```python
from build123d import *

# Parameters (mm, degrees)
F0_R     = 11.1125
F1_DEPTH = 62.0559846
F2_R     = 2.15265
F3_DEPTH = 6.35
F4_W     = 0.635
F4_H     = 0.635
F6_R     = 11.7475
F6_R_2   = 11.1125
F7_DEPTH = 0.635


# Not quite as in the source:
# - an extrude ends at something that could not be found from the text; its depth is read off the source's solid


with BuildPart() as f1:
    # F0 (on Top) → F1 (new body)
    with BuildSketch(Plane.XY):
        with BuildLine():
            ThreePointArc((14.2875, 0), (0, 14.2875), (-14.2875, 0))
            Line((-14.2875, 0), (-14.2875, -7.9375))
            Line((-14.2875, -7.9375), (-23.8125, -7.9375))
            Line((-23.8125, -7.9375), (-23.8125, -14.2875))
            Line((-23.8125, -14.2875), (23.8125, -14.2875))
            Line((23.8125, -14.2875), (23.8125, -7.9375))
            Line((23.8125, -7.9375), (14.2875, -7.9375))
            Line((14.2875, -7.9375), (14.2875, 0))
        make_face()
        Circle(F0_R, mode=Mode.SUBTRACT)
    extrude(amount=F1_DEPTH)

    # F2 (on face) → F3 (cut, through all)
    with BuildSketch(Plane.XZ.offset(14.2875)):
        with Locations((-19.05, 4.7625)):
            Circle(F2_R)
        with Locations((-19.05, 57.2934846)):
            Circle(F2_R)
        with Locations((19.05, 57.2934846)):
            Circle(F2_R)
        with Locations((19.05, 4.7625)):
            Circle(F2_R)
    extrude(amount=-F3_DEPTH, mode=Mode.SUBTRACT)

    # F5: sweep along a path in F5_path
    with BuildLine(Plane(origin=(23.8125, -14.2875, 62.0559846), x_dir=(0, -1, 0), z_dir=(0, 0, -1))) as f5_path:
        Line((0, 0), (0, 47.625))
        Line((0, 47.625), (-6.35, 47.625))
        Line((-6.35, 47.625), (-6.35, 38.1))
        Line((-6.35, 38.1), (-14.2875, 38.1))
        ThreePointArc((-14.2875, 38.1), (-28.575, 23.8125), (-14.2875, 9.525))
        Line((-14.2875, 9.525), (-6.35, 9.525))
        Line((-6.35, 9.525), (-6.35, 0))
        Line((-6.35, 0), (0, 0))
    # F4 (on face) → F5 (sweep, cut)
    with BuildSketch(Plane(origin=(-23.8125, 0, 0), x_dir=(0, -1, 0), z_dir=(-1, 0, 0))):
        with Locations((13.97, 61.7384846)):
            Rectangle(F4_W, F4_H)
    sweep(path=f5_path.line, transition=Transition.RIGHT, mode=Mode.SUBTRACT)

    # F6 (on face) → F7 (cut, through all)
    with BuildSketch(Plane.XY.offset(62.0559846)):
        Circle(F6_R)
        Circle(F6_R_2, mode=Mode.SUBTRACT)
    extrude(amount=-F7_DEPTH, mode=Mode.SUBTRACT)


solid = f1.part
```
Here's how the part is built. I have some questions about the finished solid (model axes, mm). A direction names the side the tool comes from. Coordinates: 2 decimals unless noted, no trailing zeros. Order: outer loops, then holes, each group sorted by start corner. A loop starts at its lowest first (then second) coordinate and runs counter-clockwise, first axis right, second up.
1) Imagine slicing it at C-C on x = 0. List the corners of the cut face in (y, z) for me.
2) I need wall thicknesses on line 1 (Z direction, x = 19.05, y = -12.25); line 2 (Y direction, x = -18, z = 45.5); line 3 (X direction, y = -9.25, z = 58.5). Which ranges of each line are inside material? Lowest first, please.
3) Will these pins go through, and if not, where does the flat tip stop? pin 1 (4 mm diameter, centred on y = 3.5, z = 11.5, fed in from +X); pin 2 (5 mm diameter, centred on x = 20.5, z = 36.5, fed in from +Y); pin 3 (0.7 mm diameter, centred on x = 18.5, z = 62, fed in from +Y).
4) Imagine slicing it at D-D on y = -10.25. List the corners of the cut face in (x, z) for me, and give its area (3 significant figures).
5) Which directions (+Z, -Z, +X, -X, +Y, -Y) give clear straight access to the entire face, cutting with the end or side of a thin tool? Please do faces 1 (the face through (-19, -7.938, 30)), 2 (the face through (2, -12, 0)), 3 (the face through (14.288, -4, 30)), 4 (the face through (-2.547, -11.468, 61.743)).
6) Imagine slicing it at A-A on x = 19.05. List the corners of the cut face in (y, z) for me.
7) Imagine slicing it at B-B on z = 29. List the corners of the cut face in (x, y) for me (1 decimal), and give its area (3 significant figures).
8) We'd pull the mould along Y, two halves only. Please class faces 5 (the face through (-7, -9, 61.421)), 6 (the face through (-14.288, -4, 30)), 7 (the face through (-0.3, 13.65, 61.73)), 8 (the face through (0, -14.288, 30)): +Y half, -Y half, draft (parallel to the pull), parting line (faces both ways), or undercut.
Response values:
1. outline: (-14.29, 0) - (-11.11, 0) - (-11.11, 61.42) - (-11.75, 61.42) - (-11.75, 62.06) - (-13.65, 62.06) - (-13.65, 61.42) - (-14.29, 61.42) - close; (11.11, 0) - (14.29, 0) - (14.29, 61.42) - (13.65, 61.42) - (13.65, 62.06) - (11.75, 62.06) - (11.75, 61.42) - (11.11, 61.42) - close
2. line 1: z = 0 to 2.61, 6.92 to 55.14, 59.45 to 62.06
2. line 2: y = -14.29 to -7.94
2. line 3: x = -23.81 to -20.83, -17.27 to -6.16, 6.16 to 17.27, 20.83 to 23.81
3. pin 1: stops at x = 14.21
3. pin 2: stops at y = -7.94
3. pin 3: stops at y = -8.57
4. outline: (-23.81, 0) - (-4.29, 0) - (-4.29, 61.42) - (-5.74, 61.42) - (-5.74, 62.06) - (-23.18, 62.06) - (-23.18, 61.42) - (-23.81, 61.42) - close; (4.29, 0) - (23.81, 0) - (23.81, 61.42) - (23.18, 61.42) - (23.18, 62.06) - (5.74, 62.06) - (5.74, 61.42) - (4.29, 61.42) - close; hole circle Ø4.31 at (-19.05, 4.76); hole circle Ø4.31 at (-19.05, 57.29); hole circle Ø4.31 at (19.05, 4.76); hole circle Ø4.31 at (19.05, 57.29)
4. area: 2,360 mm2
5. face 1: +Z, -Z, -X, +Y
5. face 2: -Z, +X, -X, +Y, -Y
5. face 3: +Z, -Z, +X, +Y
5. face 4: +Z
6. outline: (-14.29, 0) - (-7.94, 0) - (-7.94, 2.61) - (-14.29, 2.61) - close; (-14.29, 6.92) - (-7.94, 6.92) - (-7.94, 55.14) - (-14.29, 55.14) - close; (-14.29, 59.45) - (-7.94, 59.45) - (-7.94, 61.42) - (-8.57, 61.42) - (-8.57, 62.06) - (-13.65, 62.06) - (-13.65, 61.42) - (-14.29, 61.42) - close
7. outline: (-23.8, -14.3) - (23.8, -14.3) - (23.8, -7.9) - (14.3, -7.9) - (14.3, 0) arc R14.3 ccw to (-14.3, 0) - (-14.3, -7.9) - (-23.8, -7.9) - close; hole circle Ø22.2 at (0, 0)
7. area: 462 mm2
8. face 5: undercut
8. face 6: draft
8. face 7: +Y half
8. face 8: -Y half
